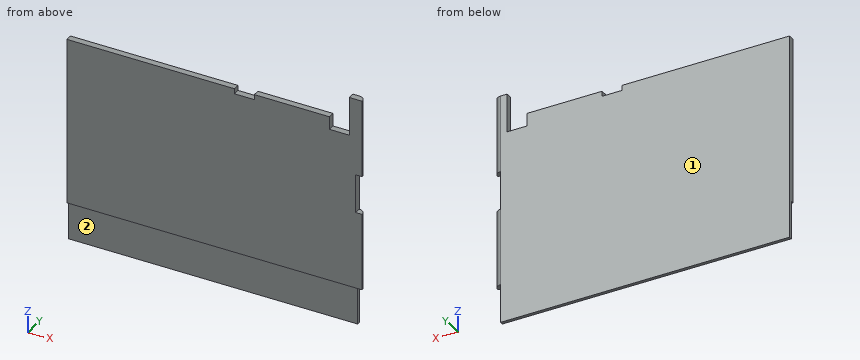
from build123d import *

# Parameters (mm, degrees)
SKETCH_1_W          = 5
SKETCH_1_H          = 60
SKETCH_1_W_2        = 30
SKETCH_1_H_2        = 5
SKETCH_1_W_3        = 15
EXTRUDE_1_DEPTH     = 5
FILLET_1_R          = 5
SKETCH_2_W          = 245
SKETCH_2_H          = 155
CUT_EXTRUDE_1_DEPTH = 5
SKETCH_3_W          = 30
SKETCH_3_H          = 2.5
CUT_EXTRUDE_2_DEPTH = 365.296775248


with BuildPart() as part:
    # 草圖1 → 填料-伸長1 (new body)
    with BuildSketch(Plane(origin=(0, 0, 0), x_dir=(1, 0, 0), z_dir=(0, 1, 0))):
        Polygon((198.746286718, -286.464902661), (198.746286718, -256.464902661), (183.246286718, -256.464902661), (183.246286718, -266.464902661), (124.746286718, -266.464902661), (124.746286718, -262.464902661), (109.246286718, -262.464902661), (109.246286718, -266.464902661), (-21.253713282, -266.464902661), (-21.253713282, 38.535097339), (-36.253713282, 38.535097339), (-36.253713282, 43.535097339), (203.746286718, 43.535097339), (203.746286718, -286.464902661), align=None)
        with Locations((206.246286718, -256.464902661)):
            Rectangle(SKETCH_1_W, SKETCH_1_H)
        with Locations((206.246286718, 13.535097339)):
            Rectangle(SKETCH_1_W, SKETCH_1_H)
        with Locations((188.746286718, 46.035097339)):
            Rectangle(SKETCH_1_W_2, SKETCH_1_H_2)
        with Locations((-21.253713282, 46.035097339)):
            Rectangle(SKETCH_1_W_2, SKETCH_1_H_2)
        with Locations((91.246286718, 46.035097339)):
            Rectangle(SKETCH_1_W_3, SKETCH_1_H_2)
        with Locations((76.246286718, 46.035097339)):
            Rectangle(SKETCH_1_W_3, SKETCH_1_H_2)
        with Locations((206.246286718, -166.464902661)):
            Rectangle(SKETCH_1_W, SKETCH_1_H)
        with Locations((206.246286718, -76.464902661)):
            Rectangle(SKETCH_1_W, SKETCH_1_H)
    extrude(amount=EXTRUDE_1_DEPTH)

    # 圓角1
    fillet_1_edges = [part.edges().sort_by_distance(p)[0] for p in [
        (208.746286718, 5, -13.535097339),
        (208.746286718, 5, 76.464902661),
        (208.746286718, 5, 166.464902661),
        (208.746286718, 5, 256.464902661),
    ]]
    fillet(fillet_1_edges, radius=FILLET_1_R - 0.0001)  # a hair under: the kernel refuses the full size

    # 草圖2 → 除料-伸長1 (cut)
    with BuildSketch(Plane(origin=(0, 5, 0), x_dir=(1, 0, 0), z_dir=(0, 1, 0))):
        with Locations((86.246286718, -28.964902661)):
            Rectangle(SKETCH_2_W, SKETCH_2_H)
    extrude(amount=-CUT_EXTRUDE_1_DEPTH, mode=Mode.SUBTRACT)

    # 草圖3 → 除料-伸長2 (cut, through all)
    with BuildSketch(Plane(origin=(203.746286718, 0, 0), x_dir=(0, 0, -1), z_dir=(1, 0, 0))):
        with Locations((-121.464902661, 1.25)):
            Rectangle(SKETCH_3_W, SKETCH_3_H)
    extrude(amount=-CUT_EXTRUDE_2_DEPTH, mode=Mode.SUBTRACT)


solid = part.part
Source: CAD feature listing. Evaluate the final solid. Frame: model axes, mm. Face numbers are marked on the shaded views. A direction names the side the tool comes from. Give positions to 0.01 mm unless a question says otherwise; leave off trailing zeros. Loops run counter-clockwise (first coordinate to the right, second up) from the corner with the lowest first, then second, coordinate; pieces in that order, holes last. Notation, with made-up numbers: (-33.5, 37.5) -> (25.5, 37.5) arc R27 cw to (25.5, 55.5) -> close; hole circle Ø8 at (-36.5, -8.75). An arc over 180 degrees is marked (long way). Use a Markdown table: item, result. Add a question column.
1) First-contact query: pin 1 (2.5 mm diameter, centred on y = 3, z = 262, fed in from +X); pin 2 (2.5 mm diameter, centred on y = 3.5, z = 207.5, fed in from +X); pin 3 (1.5 mm diameter, centred on x = 31.5, y = 3, fed in from +Z). Flat tips, straight axial feed; report the tip coordinate or a pass-through.
2) Reachability of the marked faces 1 and 2 from +Z, -Z, +X, -X, +Y, -Y: full face, straight path, thin tool, end or side. Return the list, or none.
3) Section query B-B, the plane y = 0.9. Return the cut outline in (x, z), then the cut area to 3 significant figures.
4) Section query C-C, the plane z = 204. Return the cut outline in (x, y).
5) Section query D-D, the plane x = 113. Return the cut outline in (y, z), then the cut area to 3 significant figures.
6) Line query: line 1 along Z through (x, y) = (56.5, 3.4); line 2 along Y through (x, z) = (97.5, 127.5); line 3 along X through (y, z) = (3.15, 210.5). Output: solid intervals per line, ascending. Write a range as [from, to].
7) Section query A-A, the plane x = 77. Return the cut outline in (y, z).
Numbers:
| question | item | result |
|---|---|---|
| 1 | pin 1 | stops at x = 208.43 |
| 1 | pin 2 | stops at x = 203.75 |
| 1 | pin 3 | stops at z = 266.46 |
| 2 | face 1 | +Z, -Z, +X, -X, +Y |
| 2 | face 2 | -Z, +X, -X, -Y |
| 3 | outline | (-21.25, 136.46) -> (208.66, 136.46) -> (208.66, 196.46) -> (203.75, 196.46) -> (203.75, 226.46) -> (208.66, 226.46) -> (208.66, 286.46) -> (198.75, 286.46) -> (198.75, 256.46) -> (183.25, 256.46) -> (183.25, 266.46) -> (124.75, 266.46) -> (124.75, 262.46) -> (109.25, 262.46) -> (109.25, 266.46) -> (-21.25, 266.46) -> close |
| 3 | area | 29,700 mm2 |
| 4 | outline | (-21.25, 0) -> (203.75, 0) -> (203.75, 5) -> (-21.25, 5) -> close |
| 5 | outline | (0, 136.46) -> (2.5, 136.46) -> (2.5, 106.46) -> (5, 106.46) -> (5, 262.46) -> (0, 262.46) -> close |
| 5 | area | 705 mm2 |
| 6 | line 1 | z = [106.46, 266.46] |
| 6 | line 2 | y = [2.5, 5] |
| 6 | line 3 | x = [-21.25, 203.75] |
| 7 | outline | (0, 136.46) -> (2.5, 136.46) -> (2.5, 106.46) -> (5, 106.46) -> (5, 266.46) -> (0, 266.46) -> close |
